For this review, take the finished solid that the model builds, in its own axes (mm). A direction names the side the tool comes from. Give positions to 0.01 mm unless a question says otherwise; leave off trailing zeros. Write each loop counter-clockwise with the first axis right and the second up, starting at its lowest first coordinate (ties: lowest second). Pieces come first, ordered by that corner, then holes.
1) Wall thickness on line 1 along Y through (x, z) = (25.4, 13.5); line 2 along Y through (x, z) = (0, 14.5); line 3 along Y through (x, z) = (0, 17.8): over which ranges is each line inside the solid? List them lowest first.
2) For P1, Ø8, axis at x = 25.4, y = 25.4, coming from the -Z side; P2, Ø6, axis at x = -25.4, y = -25.4, coming from the +Z side; P3, Ø6, axis at x = -25.4, y = 25.4, coming from the -Z side, all flat-tipped, find the tip position at first contact; note any pin that passes through.
3) Machinability: for faces 4 (the face through (26.772, -27.552, 9.401)), 5 (the face through (-3.1, 13.96, 5.08)), which of the approach directions +Z, -Z, +X, -X, +Y, -Y give a long, thin tool a straight path to every point of the face, cutting with its end or side? Answer none if there is none.
4) Draft analysis for pull direction X (two halves, no side actions). For faces 1 (the face through (4, -13, 11.074)), 2 (the face through (0, 31.75, 9)), 3 (the face through (29.474, 29.564, 18.94)), state which applies: pulls with the +X half, pulls with the -X half, needs draft (parallel to the pull), parting line crosses it, or undercut.
5) We need section A-A on z = 15. Give the boundary of the cut face in (x, y), and give its area (3 significant figures).
Autodesk Inventor part; units mm, degrees
ref_plane "Work Plane1" through (0, 0, 9.525) normal (0, 0, 1) x (1, 0, 0)
ref_plane "YZ Plane" through (0, 0, 0) normal (1, 0, 0) x (0, 1, 0)
ref_plane "XZ Plane" through (0, 0, 0) normal (0, 1, 0) x (-1, 0, 0)
sketch "Sketch1" plane through (0, 0, 0) normal (0, 0, 1) x (1, 0, 0)
  line L0 (-31.75, -31.75) -> (31.75, -31.75)
  line L1 (31.75, -31.75) -> (31.75, 31.75)
  line L2 (31.75, 31.75) -> (-31.75, 31.75)
  line L3 (-31.75, 31.75) -> (-31.75, -31.75)
  line L4 (-31.75, -31.75) -> (31.75, 31.75) construction
  line L5 (31.75, -31.75) -> (-31.75, 31.75) construction
  circle A0 centre (-25.4, 25.4) radius 2.5527
  circle A1 centre (25.4, 25.4) radius 2.5527
  circle A2 centre (-25.4, -25.4) radius 2.5527
  circle A3 centre (25.4, -25.4) radius 2.5527
  circle A4 centre (0, 0) radius 12.6746
  dimension "d0" = 63.5
  dimension "d1" = 63.5
  dimension "d2" = 6.35
  dimension "d5" = 50.8
  dimension "d8" = 50.8
  dimension "d11" = 5.1054
  dimension "d12" = 25.3492
extrude "Extrusion1" add sketch "Sketch1" along normal blind 19.05
fillet "Fillet1" radius 6.35 4 edges at (31.75, 31.75, 9.525) (31.75, -31.75, 9.525) (-31.75, -31.75, 9.525) (-31.75, 31.75, 9.525)
sketch "Sketch2" plane through (0, 0, 19.05) normal (0, 0, 1) x (1, 0, 0)
  circle A0 centre (0, 0) radius 14.3002
  dimension "d16" = 28.6004
extrude "Extrusion2" cut sketch "Sketch2" against normal blind 7.9756
sketch "Sketch3" plane through (0, 0, 19.05) normal (0, 0, 1) x (1, 0, 0)
  circle A0 centre (0, 0) radius 15.5702
  dimension "d19" = 31.1404
extrude "Extrusion3" cut sketch "Sketch3" against normal blind 1.6256
ref_plane "Work Plane1" through (0, 0, 9.525) normal (0, 0, 1) x (1, 0, 0)
mirror "Mirror1" about plane through (0, 0, 9.525) normal (0, 0, 1) of "Extrusion2", "Extrusion3"
chamfer "Chamfer1" distance 0.635 angle 45 16 edges at (-31.75, 0, 19.05) (-29.8901, -29.8901, 19.05) (0, -31.75, 19.05) (29.8901, -29.8901, 19.05) (31.75, 0, 19.05) (29.8901, 29.8901, 19.05) (0, 31.75, 19.05) (-29.8901, 29.8901, 19.05) (0, -31.75, 0) (29.8901, -29.8901, 0) (31.75, 0, 0) (29.8901, 29.8901, 0) (0, 31.75, 0) (-29.8901, 29.8901, 0) (-31.75, 0, 0) (-29.8901, -29.8901, 0)
chamfer "Chamfer2" distance 0.635 angle 45 6 edges at (-15.5702, 0, 19.05) (-14.3002, 0, 17.4244) (-12.6746, 0, 11.0744) (-12.6746, 0, 7.9756) (-14.3002, 0, 1.6256) (-15.5702, 0, 0)
chamfer "Chamfer3" distance 0.635 angle 45 8 edges at (-27.9527, -25.4, 19.05) (22.8473, -25.4, 19.05) (22.8473, 25.4, 19.05) (-27.9527, 25.4, 19.05) (22.8473, 25.4, 0) (22.8473, -25.4, 0) (-27.9527, -25.4, 0) (-27.9527, 25.4, 0)
properties part number "BearingBlockForPrototypePlate2"
Results list:
1. line 1: y = -31.75 to -27.95, -22.85 to 22.85, 27.95 to 31.75
1. line 2: y = -31.75 to -14.3, 14.3 to 31.75
1. line 3: y = -31.75 to -15.57, 15.57 to 31.75
2. P1: stops at z = 0
2. P2: stops at z = 18.86
2. P3: stops at z = 0.19
3. face 4: +Z, -Z
3. face 5: -Z
4. face 1: undercut
4. face 2: needs draft
4. face 3: pulls with the +X half
5. outline: (-31.75, -25.4) arc R6.35 ccw to (-25.4, -31.75) - (25.4, -31.75) arc R6.35 ccw to (31.75, -25.4) - (31.75, 25.4) arc R6.35 ccw to (25.4, 31.75) - (-25.4, 31.75) arc R6.35 ccw to (-31.75, 25.4) - close; hole circle Ø5.11 at (-25.4, -25.4); hole circle Ø5.11 at (-25.4, 25.4); hole circle Ø28.6 at (0, 0); hole circle Ø5.11 at (25.4, -25.4); hole circle Ø5.11 at (25.4, 25.4)
5. area: 3,270 mm2
